Autodesk Inventor part; units mm, degrees
ref_plane "YZ Plane" through (0, 0, 0) normal (1, 0, 0) x (0, 1, 0)
ref_plane "XZ Plane" through (0, 0, 0) normal (0, 1, 0) x (-1, 0, 0)
ref_plane "XY Plane" through (0, 0, 0) normal (0, 0, 1) x (1, 0, 0)
sketch "スケッチ1" plane through (0, 0, 0) normal (0, 1, 0) x (-1, 0, 0)
  line L0 (9.5, -9.5) -> (0, -9.5)
  line L1 (0, -9.5) -> (0, -2.5)
  line L2 (0, 0) -> (3.15, 0)
  line L3 (9.5, 0) -> (9.5, -9.5)
  line L4 (0, 0) -> (3.15, 0)
  line L5 (3.15, 0) -> (3.15, -1)
  line L6 (1.65, -2.5) -> (0, -2.5)
  line L7 (0, -2.5) -> (0, 0)
  arc A0 (1.65, -2.5) -> (3.15, -1) centre (1.65, -1) ccw
  line L8 (3.15, 0) -> (6.325, 0)
  line L9 (6.325, 0) -> (9.5, 0)
  line L10 (0, -2.5) -> (0, 0)
  line L11 (9.5, 9.5) -> (0, 9.5)
  line L12 (9.5, 0) -> (9.5, 9.5)
  line L13 (3.15, 0) -> (3.15, 1)
  line L14 (1.65, 2.5) -> (0, 2.5)
  arc A1 (3.15, 1) -> (1.65, 2.5) centre (1.65, 1) ccw
  line L15 (-9.5, -9.5) -> (0, -9.5)
  line L16 (-9.5, 0) -> (-9.5, -9.5)
  line L17 (-3.15, 0) -> (-3.15, -1)
  line L18 (-1.65, -2.5) -> (0, -2.5)
  arc A2 (-3.15, -1) -> (-1.65, -2.5) centre (-1.65, -1) ccw
  line L19 (-9.5, 9.5) -> (0, 9.5)
  line L20 (-9.5, 0) -> (-9.5, 9.5)
  line L21 (-3.15, 0) -> (-3.15, 1)
  arc A3 (-1.65, 2.5) -> (-3.15, 1) centre (-1.65, 1) ccw
  line L22 (-1.65, 2.5) -> (0, 2.5)
  point P0 (-6.325, 0)
  dimension "d2" = 1.5
  dimension "d3" = 19
  dimension "d4" = 6.3
  dimension "d5" = 5
  dimension "d6" = 19
extrude "押し出し1" add sketch "スケッチ1" along normal blind 1.4
sketch "スケッチ2" plane through (0, 1.4, 0) normal (0, 1, 0) x (1, 0, 0)
  line L0 (9.5, 9.5) -> (-9.5, 9.5)
  line L1 (0, 9.5) -> (0, 7.5)
  line L2 (0, 7.5) -> (0, 2.5)
  line L3 (0, 2.5) -> (0, 0)
  line L4 (-3.15, 7.5) -> (3.15, 7.5)
  line L5 (3.15, 7.5) -> (3.15, 2.5)
  line L6 (3.15, 2.5) -> (-3.15, 2.5)
  line L7 (-3.15, 2.5) -> (-3.15, 7.5)
  line L8 (-9.5, 9.5) -> (-9.5, -9.5)
  line L9 (-9.5, 0) -> (9.5, 0)
  line L10 (9.5, -9.5) -> (9.5, 9.5)
  line L11 (-3.15, -7.5) -> (3.15, -7.5)
  line L12 (3.15, -7.5) -> (3.15, -2.5)
  line L13 (3.15, -2.5) -> (-3.15, -2.5)
  line L14 (-3.15, -2.5) -> (-3.15, -7.5)
  dimension "d11" = 6.3
  dimension "d12" = 2.5
  dimension "d13" = 5
extrude "押し出し2" add sketch "スケッチ2" along normal blind 1.6 contours L4 L5 L6 L2 | L2 L6 L7 L4 | L14 L13 L12 L11
fillet "フィレット1" radius 1.5 8 edges at (-3.15, 2.2, -2.5) (-3.15, 2.2, 7.5) (3.15, 2.2, 7.5) (3.15, 2.2, 2.5) (-3.15, 2.2, 2.5) (3.15, 2.2, -2.5) (3.15, 2.2, -7.5) (-3.15, 2.2, -7.5)
sketch "スケッチ3" plane through (0, 1.4, 0) normal (0, 1, 0) x (1, 0, 0)
  arc A0 (-1.65, 7.5) -> (-3.15, 6) centre (-1.65, 6) ccw
  line L0 (-3.15, 6) -> (-3.15, 4)
  arc A1 (-3.15, 4) -> (-1.65, 2.5) centre (-1.65, 4) ccw
  line L1 (-1.65, 2.5) -> (1.65, 2.5)
  arc A2 (1.65, 2.5) -> (3.15, 4) centre (1.65, 4) ccw
  line L2 (3.15, 4) -> (3.15, 6)
  arc A3 (3.15, 6) -> (1.65, 7.5) centre (1.65, 6) ccw
  line L3 (1.65, 7.5) -> (-1.65, 7.5)
  arc A4 (-1.65, -2.5) -> (-3.15, -4) centre (-1.65, -4) ccw
  line L4 (-3.15, -4) -> (-3.15, -6)
  arc A5 (-3.15, -6) -> (-1.65, -7.5) centre (-1.65, -6) ccw
  line L5 (-1.65, -7.5) -> (1.65, -7.5)
  arc A6 (1.65, -7.5) -> (3.15, -6) centre (1.65, -6) ccw
  line L6 (3.15, -6) -> (3.15, -4)
  arc A7 (3.15, -4) -> (1.65, -2.5) centre (1.65, -4) ccw
  line L7 (1.65, -2.5) -> (-1.65, -2.5)
  line L8 (-3.15, 5) -> (-9.5, 5)
  line L9 (-9.5, 9.5) -> (-9.5, -9.5)
  line L10 (-9.5, 0) -> (0, 0)
  line L11 (0, 0) -> (0, 9.5)
  line L12 (9.5, 9.5) -> (-9.5, 9.5)
  point P0 (-6.325, 5)
  point P1 (-6.325, -5)
  point P2 (6.325, 5)
  point P3 (6.325, -5)
hole "穴1" at (-6.325, 1.4, -5) at (-6.325, 1.4, 5) at (6.325, 1.4, -5) at (6.325, 1.4, 5) direction (0, -1, 0) diameter 1.567 end through all
sketch "スケッチ4" plane through (0, 0, 0) normal (0, -1, 0) x (1, 0, 0)
  line L0 (-2.5, 9.5) -> (2.5, 9.5)
  line L1 (2.5, 9.5) -> (2.5, 6.5)
  line L2 (2.5, 6.5) -> (-2.5, 6.5)
  line L3 (-2.5, 6.5) -> (-2.5, 9.5)
  line L4 (-9.5, 9.5) -> (9.5, 9.5)
  point P0 (0, 0)
  point P1 (0, 9.5)
  dimension "d24" = 5
  dimension "d25" = 3
extrude "押し出し3" cut sketch "スケッチ4" against normal blind 1.6
sketch "スケッチ5" plane through (-2.5, 0, 9.5) normal (1, 0, 0) x (0, 0, -1)
  line L0 (2.2641, 1.4) -> (2.2641, 1.6)
  line L1 (0, 1.4) -> (2.2641, 1.4)
  line L2 (0, 0) -> (0, 1.4)
  line L3 (3, 0) -> (0, 0)
  line L4 (3, 0) -> (3, 1.6)
  line L5 (3, 1.6) -> (2.2641, 1.6)
  spline S0 degree 2 poles (3, 0) (2.1867, 1.089) (0, 1.4) knots 0 0 0 1 1 1
  point P0 (9.5, 0)
  point P1 (2.0329, 0.8)
extrude "押し出し4" add sketch "スケッチ5" along normal up to surface (5 mm away) contours L0 L5 L4 S0 L1
sketch "スケッチ6" plane through (0, 1.6, 0) normal (0, -1, 0) x (1, 0, 0)
  line L0 (-2.5, 7.2359) -> (2.5, 7.2359)
  arc A0 (2.5, 7.2359) -> (1.65, 7.5) centre (1.65, 6) ccw
  line L1 (-1.65, 7.5) -> (1.65, 7.5)
  arc A1 (-1.65, 7.5) -> (-2.5, 7.2359) centre (-1.65, 6) ccw
  point P0 (0, 0)
extrude "押し出し5" add sketch "スケッチ6" along normal up to surface (0.2 mm away)
fillet "フィレット2" radius 0.5 2 edges at (-2.5, 0.8945, 7.6566) (2.5, 0.8945, 7.6566)
properties part number "sensorbar"
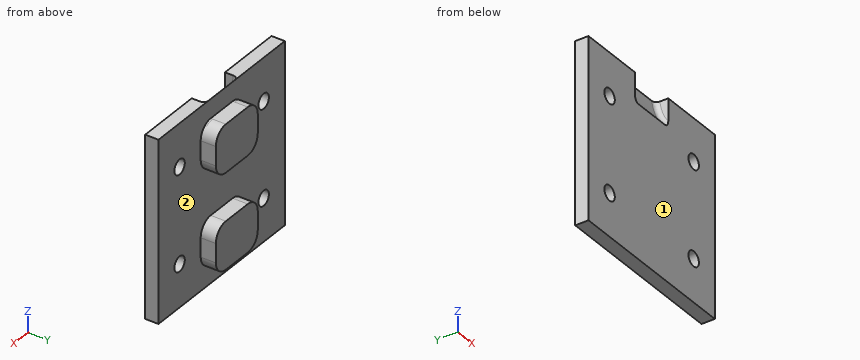
Could you check a few things on this model? Use its own coordinates, in mm. Face numbers are marked on the shaded views. A direction names the side the tool comes from. Give positions to 0.01 mm unless a question says otherwise; leave off trailing zeros. Loops run counter-clockwise (first coordinate to the right, second up) from the corner with the lowest first, then second, coordinate; pieces in that order, holes last. Notation, with made-up numbers: (43, 79.5) - (83, 79.5) arc R16 cw to (83, 93.5) - close; hole circle Ø11 at (16, -3.75). An arc over 180 degrees is marked (long way). Answer in a Markdown table with one row per item. Add a question column.
Q1. If we section it at D-D (z = -0.75): List the corners of the cut face in (x, y) for me.
Q2. If we section it at B-B (z = -5): List the corners of the cut face in (x, y) for me, plus the area to 3 significant figures.
Q3. Please list where these lines run through material, in increasing order: L1, parallel to X at y = 0.6, z = -5; L2, parallel to Z at x = -1.75, y = 1.95; L3, parallel to Y at x = 5.75, z = -7.25. Write a range as from..to.
Q4. If we section it at A-A (y = 2.5): List the corners of the cut face in (x, z) for me, plus the area to 3 significant figures.
Q5. If we section it at C-C (x = 4.5): List the corners of the cut face in (y, z) for me, plus the area to 3 significant figures.
Q6. For pin 1 (0.8 mm diameter, centred on x = -1, y = 2, fed in from +Z); pin 2 (1.3 mm diameter, centred on x = -6.325, z = 5, fed in from +Y); pin 3 (1.5 mm diameter, centred on y = 2.5, z = 5, fed in from -X); pin 4 (0.5 mm diameter, centred on x = -0.5, y = 2, fed in from -Z), each with a flat end and sliding along its axis, tell me the tip position at first contact or that it passes through.
Q7. Which directions (+Z, -Z, +X, -X, +Y, -Y) give clear straight access to the entire face, cutting with the end or side of a thin tool? Please do the marked faces 1 and 2.
The answers:
| question | item | result |
|---|---|---|
| 1 | outline | (-9.5, 0) - (9.5, 0) - (9.5, 1.4) - (-9.5, 1.4) - close |
| 2 | outline | (-9.5, 0) - (-7.11, 0) - (-7.11, 1.4) - (-9.5, 1.4) - close; (-5.54, 0) - (5.54, 0) - (5.54, 1.4) - (3.15, 1.4) - (3.15, 3) - (-3.15, 3) - (-3.15, 1.4) - (-5.54, 1.4) - close; (7.11, 0) - (9.5, 0) - (9.5, 1.4) - (7.11, 1.4) - close |
| 2 | area | 32.3 mm^2 |
| 3 | L1 | x = -9.5..-7.11, -5.54..5.54, 7.11..9.5 |
| 3 | L2 | z = -7.5..-2.5, 2.5..7.5 |
| 3 | L3 | y = 0..1.4 |
| 4 | outline | (-3.15, -6) arc R1.5 ccw to (-1.65, -7.5) - (1.65, -7.5) arc R1.5 ccw to (3.15, -6) - (3.15, -4) arc R1.5 ccw to (1.65, -2.5) - (-1.65, -2.5) arc R1.5 ccw to (-3.15, -4) - close; (-3.15, 4) arc R1.5 ccw to (-1.65, 2.5) - (1.65, 2.5) arc R1.5 ccw to (3.15, 4) - (3.15, 6) arc R1.5 ccw to (1.65, 7.5) - (-1.65, 7.5) arc R1.5 ccw to (-3.15, 6) - close |
| 4 | area | 59.1 mm^2 |
| 5 | outline | (0, -9.5) - (1.4, -9.5) - (1.4, 9.5) - (0, 9.5) - close |
| 5 | area | 26.6 mm^2 |
| 6 | pin 1 | stops at z = 7.5 |
| 6 | pin 2 | passes through |
| 6 | pin 3 | stops at x = -3.15 |
| 6 | pin 4 | stops at z = -7.5 |
| 7 | face 1 | +Z, -Z, +X, -X, -Y |
| 7 | face 2 | +Y |
